Here's how the part is built. I have some questions about the finished solid (model axes, mm). Face numbers are marked on the shaded views. Give positions to 0.01 mm unless a question says otherwise; leave off trailing zeros. Order: outer loops, then holes, each group sorted by start corner. A loop starts at its lowest first (then second) coordinate and runs counter-clockwise, first axis right, second up. Notation, with made-up numbers: (-16.5, -31) -> (42.5, -31) arc R5 cw to (42.5, -23) -> close; hole circle Ø4 at (-33, -11). An arc over 180 degrees is marked (long way). Write each question's results on one line, items separated by ' | '. Start each with the question number.
Q1. Thinking about a two-plate mould opening in X: for the marked faces 1 and 2, which applies, pulls with the +X half, pulls with the -X half, needs draft (parallel to the pull), parting line crosses it, or undercut?
Q2. I need wall thicknesses on line 1 along Y through (x, z) = (1.7, -115.5) (3 decimals); line 2 along Y through (x, z) = (1.15, -175); line 3 along Y through (x, z) = (2.5, 0). Which ranges of each line are inside material? Lowest first, please. Write a range as [from, to].
Q3. Imagine slicing it at C-C, the plane x = 0.8. State how many separate pieces and enclosed holes the cut face has, then the cut area to 3 significant figures.
Q4. Imagine slicing it at A-A, the plane y = -220. Please give me the cut outline in (x, z) (3 decimals).
Q5. Imagine slicing it at B-B, the plane z = -115.5. Please give me the cut outline in (x, y) (3 decimals).
```python
from build123d import *

# Parameters (mm, degrees)
SKETCH1_W           = 500
SKETCH1_H           = 375
SKETCH1_R           = 2.8
BOSS_EXTRUDE1_DEPTH = 3.175
SKETCH2_R           = 9.525
CUT_EXTRUDE1_DEPTH  = 313.516128584
CUT_EXTRUDE2_DEPTH  = 313.516128584
SKETCH5_R           = 1.7
CUT_EXTRUDE3_DEPTH  = 313.516128584
SKETCH6_W           = 21.5
SKETCH6_H           = 26
CUT_EXTRUDE4_DEPTH  = 313.516128584


with BuildPart() as part:
    # Sketch1 → Boss-Extrude1 (new body)
    with BuildSketch(Plane.YZ):
        Rectangle(SKETCH1_W, SKETCH1_H)
        with Locations(Location((-237.5, 175, 0), (0, 0, 270))):
            Circle(SKETCH1_R, mode=Mode.SUBTRACT)
        with Locations(Location((237.5, 175, 0), (0, 0, 270))):
            Circle(SKETCH1_R, mode=Mode.SUBTRACT)
        with Locations(Location((237.5, -175, 0), (0, 0, 270))):
            Circle(SKETCH1_R, mode=Mode.SUBTRACT)
        with Locations(Location((-237.5, -175, 0), (0, 0, 270))):
            Circle(SKETCH1_R, mode=Mode.SUBTRACT)
        with Locations(Location((-237.5, 0, 0), (0, 0, 270))):
            Circle(SKETCH1_R, mode=Mode.SUBTRACT)
        with Locations(Location((0, 175, 0), (0, 0, 270))):
            Circle(SKETCH1_R, mode=Mode.SUBTRACT)
        with Locations(Location((237.5, 0, 0), (0, 0, 270))):
            Circle(SKETCH1_R, mode=Mode.SUBTRACT)
        with Locations(Location((0, -175, 0), (0, 0, 270))):
            Circle(SKETCH1_R, mode=Mode.SUBTRACT)
    extrude(amount=BOSS_EXTRUDE1_DEPTH)

    # Sketch2 → Cut-Extrude1 (cut, through all)
    with BuildSketch(Plane.YZ.offset(3.175)):
        with Locations(Location((-220, -115.5, 0), (0, 0, 270))):
            Circle(SKETCH2_R)
        with Locations(Location((-193, -142.5, 0), (0, 0, 270))):
            Circle(SKETCH2_R)
        with Locations(Location((-136, -115.5, 0), (0, 0, 270))):
            Circle(SKETCH2_R)
        with Locations(Location((-109, -142.5, 0), (0, 0, 270))):
            Circle(SKETCH2_R)
        with Locations(Location((-52, -115.5, 0), (0, 0, 270))):
            Circle(SKETCH2_R)
        with Locations(Location((-25, -142.5, 0), (0, 0, 270))):
            Circle(SKETCH2_R)
        with Locations(Location((32, -115.5, 0), (0, 0, 270))):
            Circle(SKETCH2_R)
        with Locations(Location((59, -142.5, 0), (0, 0, 270))):
            Circle(SKETCH2_R)
        with Locations(Location((116, -115.5, 0), (0, 0, 270))):
            Circle(SKETCH2_R)
        with Locations(Location((143, -142.5, 0), (0, 0, 270))):
            Circle(SKETCH2_R)
    extrude(amount=-CUT_EXTRUDE1_DEPTH, mode=Mode.SUBTRACT)

    # Sketch4 → Cut-Extrude2 (cut, through all)
    with BuildSketch(Plane.YZ.offset(3.175)):
        Polygon((210, -12.5), (183, -12.5), (183, 11.122), (190.112, 18.234), (202.888, 18.234), (210, 11.122), align=None)
    extrude(amount=-CUT_EXTRUDE2_DEPTH, mode=Mode.SUBTRACT)

    # Sketch5 → Cut-Extrude3 (cut, through all)
    with BuildSketch(Plane.YZ.offset(3.175)):
        with Locations(Location((178.593, 2.9, 0), (0, 0, 270))):
            Circle(SKETCH5_R)
        with Locations(Location((214.407, 2.9, 0), (0, 0, 270))):
            Circle(SKETCH5_R)
    extrude(amount=-CUT_EXTRUDE3_DEPTH, mode=Mode.SUBTRACT)

    # Sketch6 → Cut-Extrude4 (cut, through all)
    with BuildSketch(Plane.YZ.offset(3.175)):
        with Locations((196.5, 51.234)):
            Rectangle(SKETCH6_W, SKETCH6_H)
    extrude(amount=-CUT_EXTRUDE4_DEPTH, mode=Mode.SUBTRACT)


solid = part.part
```
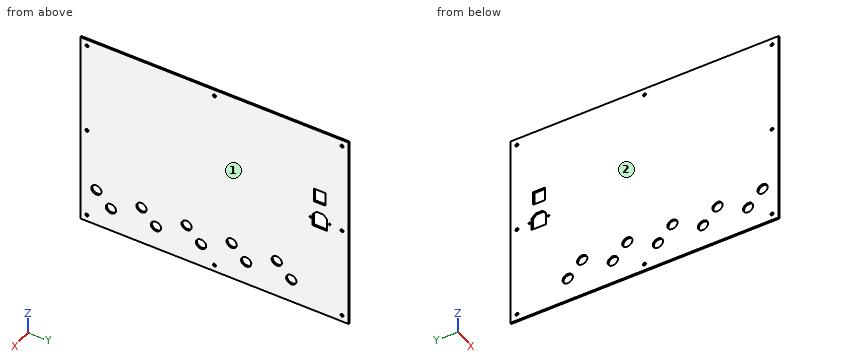
Geometry check:
1) face 1: pulls with the +X half | face 2: pulls with the -X half
2) line 1: [-250, -229.525], [-210.475, -145.525], [-126.475, -61.525], [-42.475, 22.475], [41.525, 106.475], [125.525, 250] | line 2: [-250, -240.3], [-234.7, -2.8], [2.8, 234.7], [240.3, 250] | line 3: [-250, -240.3], [-234.7, 183], [210, 234.7], [240.3, 250]
3) separate pieces: 1 | enclosed holes: 22 | area: 183,000 mm²
4) outline: (0, -187.5) -> (3.175, -187.5) -> (3.175, -125.025) -> (0, -125.025) -> close; (0, -105.975) -> (3.175, -105.975) -> (3.175, 187.5) -> (0, 187.5) -> close
5) outline: (0, -250) -> (3.175, -250) -> (3.175, -229.525) -> (0, -229.525) -> close; (0, -210.475) -> (3.175, -210.475) -> (3.175, -145.525) -> (0, -145.525) -> close; (0, -126.475) -> (3.175, -126.475) -> (3.175, -61.525) -> (0, -61.525) -> close; (0, -42.475) -> (3.175, -42.475) -> (3.175, 22.475) -> (0, 22.475) -> close; (0, 41.525) -> (3.175, 41.525) -> (3.175, 106.475) -> (0, 106.475) -> close; (0, 125.525) -> (3.175, 125.525) -> (3.175, 250) -> (0, 250) -> close
